Model file for the job. Use its own axes, mm. A direction names the side the tool comes from. Give positions to 0.01 mm unless a question says otherwise; leave off trailing zeros. Loops run counter-clockwise (first coordinate to the right, second up) from the corner with the lowest first, then second, coordinate; pieces in that order, holes last. Notation, with made-up numbers: M 76.5,29.25 L 103.5,29.25 A26 ccw 103.5,45.25 Z; hole C 19,61.5 d3. An arc over 180 degrees is marked long. Answer in a Markdown table with one row per item.
```python
from build123d import *

# Parameters (mm, degrees)
F0_W     = 6.35
F0_H     = 3.175
F0_H_2   = 6.35
F0_W_2   = 13.335
F1_DEPTH = 15.24
F2_R     = 3.175
F3_R     = 6.35
F4_R     = 9.525
F5_R     = 12.7


with BuildPart() as f1:
    # F0 (on Top) → F1 (new body)
    with BuildSketch(Plane.XY):
        Polygon((-16.51, 15.875), (-3.175, 15.875), (3.175, 15.875), (16.51, 15.875), (16.51, 22.225), (-16.51, 22.225), align=None)
        with Locations((0, 14.2875)):
            Rectangle(F0_W, F0_H)
        with Locations((0, 9.525)):
            Rectangle(F0_W, F0_H_2)
        with Locations((-9.8425, 9.525)):
            Rectangle(F0_W_2, F0_H_2)
        with Locations((9.8425, 9.525)):
            Rectangle(F0_W_2, F0_H_2)
        with Locations((0, 4.7625)):
            Rectangle(F0_W, F0_H)
        Rectangle(F0_W, F0_H_2)
        with Locations((9.8425, 0)):
            Rectangle(F0_W_2, F0_H_2)
        with Locations((-9.8425, 0)):
            Rectangle(F0_W_2, F0_H_2)
        with Locations((0, -4.7625)):
            Rectangle(F0_W, F0_H)
        Polygon((-3.175, -10.1355769231), (-3.175, -6.35), (-16.51, -6.35), (-16.51, -12.7), align=None)
        Polygon((3.175, -6.35), (-3.175, -6.35), (-3.175, -10.1355769231), (3.175, -8.9144230769), align=None)
        Polygon((16.51, -12.7), (16.51, -6.35), (3.175, -8.9144230769), (3.175, -12.7), align=None)
        with Locations((0, -14.2875)):
            Rectangle(F0_W, F0_H)
        Polygon((3.175, -15.875), (-3.175, -15.875), (-16.51, -15.875), (-16.51, -22.225), (16.51, -15.875), align=None)
        Polygon((3.175, -8.9144230769), (-3.175, -10.1355769231), (-3.175, -12.7), (3.175, -12.7), align=None)
        Polygon((-3.175, -12.7), (-3.175, -10.1355769231), (-16.51, -12.7), align=None)
        Polygon((16.51, -6.35), (3.175, -6.35), (3.175, -8.9144230769), align=None)
        Polygon((16.51, -22.225), (16.51, -15.875), (-16.51, -22.225), align=None)
    extrude(amount=F1_DEPTH)

    # F2
    f2_edges = [f1.edges().sort_by_distance(p)[0] for p in [
        (-16.51, -19.05, 0),
        (16.51, -19.05, 0),
    ]]
    fillet(f2_edges, radius=F2_R)

    # F3
    f3_edges = [f1.edges().sort_by_distance(p)[0] for p in [
        (-16.51, -9.525, 0),
        (16.51, -9.525, 0),
    ]]
    fillet(f3_edges, radius=F3_R)

    # F4
    f4_edges = [f1.edges().sort_by_distance(p)[0] for p in [
        (-16.51, 0, 0),
        (16.51, 0, 0),
    ]]
    fillet(f4_edges, radius=F4_R)

    # F5
    f5_edges = [f1.edges().sort_by_distance(p)[0] for p in [
        (16.51, 9.525, 0),
        (-16.51, 9.525, 0),
    ]]
    fillet(f5_edges, radius=F5_R)


solid = f1.part
```
Q1. Saw through at A-A (x = -9). Give the cut face in (y, z) (3 decimals), and give its area (3 significant figures).
Reported:
| item | result |
|---|---|
| outline | M -22.225,0 L -15.875,0 L -15.875,15.24 L -22.225,15.24 Z; M -12.7,0 L -6.35,0 L -6.35,15.24 L -12.7,15.24 Z; M -3.175,0.216 L 3.175,0.216 L 3.175,15.24 L -3.175,15.24 Z; M 6.35,1.109 L 12.7,1.109 L 12.7,15.24 L 6.35,15.24 Z; M 15.875,0 L 22.225,0 L 22.225,15.24 L 15.875,15.24 Z |
| area | 475 mm² |
Q2. 3-axis set-ups, long thin cutter, end or side, ignore diameter. For faces 1 (the face through (-15.6, -19.09, 0.95)), 2 (the face through (3.175, 14, 8)), 3 (the face through (-10, -6.35, 8)): which of +Z, -Z, +X, -X, +Y, -Y reach the whole face in a straight line?
Reported:
| item | result |
|---|---|
| face 1 | -Z, -X, -Y |
| face 2 | +Z, -Z, +X |
| face 3 | +Z, -Z, -X |
Q3. Saw through at C-C (x = 8). Give the cut face in (y, z) (3 decimals).
Reported:
| item | result |
|---|---|
| outline | M -22.225,0 L -15.875,0 L -15.875,15.24 L -22.225,15.24 Z; M -12.7,0 L -6.35,0 L -6.35,15.24 L -12.7,15.24 Z; M -3.175,0.054 L 3.175,0.054 L 3.175,15.24 L -3.175,15.24 Z; M 6.35,0.711 L 12.7,0.711 L 12.7,15.24 L 6.35,15.24 Z; M 15.875,0 L 22.225,0 L 22.225,15.24 L 15.875,15.24 Z |
Q4. Saw through at B-B (y = 11). Give the cut face in (x, z).
Reported:
| item | result |
|---|---|
| outline | M -16.51,12.7 A12.7 ccw -3.81,0 L 3.81,0 A12.7 ccw 16.51,12.7 L 16.51,15.24 L -16.51,15.24 Z |
Q5. Probe probe 1 along Y at (x, z) = (13.5, 8.25) (3 decimals); probe 2 along Y at (x, z) = (-12.5, 2) (3 decimals). List the from-to ranges inside material, lowest first.
Reported:
| item | result |
|---|---|
| probe 1 | -22.225 to -15.875, -12.7 to -6.35, -3.175 to 3.175, 6.35 to 12.7, 15.875 to 22.225 |
| probe 2 | -22.225 to -15.875, -12.7 to -6.35, -3.175 to 3.175, 15.875 to 22.225 |
Q6. Mould opens along Y. For faces 4 (the face through (-16.51, 9, 14)), 5 (the face through (10, 15.875, 8)) say: released by +Y, released by -Y, zero draft, split by the parting line, or undercut.
Reported:
| item | result |
|---|---|
| face 4 | zero draft |
| face 5 | undercut |
Q7. Drop flat-ended pins along their axis: pin 1 (8 mm diameter, centred on y = 10.5, z = 4.5, fed in from -X); pin 2 (3.5 mm diameter, centred on y = 4.5, z = 8, fed in from +X); pin 3 (2.5 mm diameter, centred on y = 5, z = 5, fed in from -X) (3 decimals). Give the stop position or say it passes through.
Reported:
| item | result |
|---|---|
| pin 1 | x = -15.8 |
| pin 2 | x = 16.5 |
| pin 3 | x = -3.175 |
Q8. Saw through at D-D (y = -2). Give the cut face in (x, z) (3 decimals).
Reported:
| item | result |
|---|---|
| outline | M -16.51,9.525 A9.525 ccw -6.985,0 L 6.985,0 A9.525 ccw 16.51,9.525 L 16.51,15.24 L -16.51,15.24 Z |
